Geometry check sheet. Reference: the model listing, model coordinates, mm. A direction names the side the tool comes from. Round coordinates to 2 decimals unless told otherwise and drop trailing zeros. Order: outer loops, then holes, each group sorted by start corner. A loop starts at its lowest first (then second) coordinate and runs counter-clockwise, first axis right, second up. Notation, with made-up numbers: (-5, 29.5) -> (38, 29.5) arc R11 cw to (38, 35.5) -> close; hole circle Ø10 at (-3.5, 23). An arc over 180 degrees is marked (long way). Answer as a JSON object with one key per item and string values. Group by question number.
from build123d import *

# Parameters (mm, degrees)
F0_R     = 10
F1_DEPTH = 7.5
F2_R     = 10
F3_R     = 10
F4_R     = 15
F5_R     = 15


with BuildPart() as f1:
    # F0 (on Front) → F1 (new body, symmetric)
    with BuildSketch(Plane.XZ):
        with BuildLine():
            ThreePointArc((-19.027325, -11.591323), (-14.510885, -6.560614), (-12.878518, 0))
            ThreePointArc((-12.878518, 0), (-14.510885, 6.560614), (-19.027325, 11.591323))
            ThreePointArc((-19.027325, 11.591323), (-40.878518, 0), (-19.027325, -11.591323))
        make_face()
        with Locations((-26.878518, 0)):
            Circle(F0_R, mode=Mode.SUBTRACT)
        with BuildLine():
            Line((54.121482, 0), (-12.878518, 0))
            ThreePointArc((-12.878518, 0), (-14.510885, -6.560614), (-19.027325, -11.591323))
            Line((-19.027325, -11.591323), (63.640685, -21.482518))
            ThreePointArc((63.640685, -21.482518), (56.607871, -11.748551), (54.121482, 0))
        make_face()
        with BuildLine():
            ThreePointArc((-19.027325, 11.591323), (-14.510885, 6.560614), (-12.878518, 0))
            Line((-12.878518, 0), (54.121482, 0))
            ThreePointArc((54.121482, 0), (56.607871, 11.748551), (63.640685, 21.482518))
            Line((63.640685, 21.482518), (-19.027325, 11.591323))
        make_face()
        with BuildLine():
            ThreePointArc((63.640685, 21.482518), (56.607871, 11.748551), (54.121482, 0))
            ThreePointArc((54.121482, 0), (56.607871, -11.748551), (63.640685, -21.482518))
            ThreePointArc((63.640685, -21.482518), (94.870033, -26.513611), (112.121482, 0))
            ThreePointArc((112.121482, 0), (94.870033, 26.513611), (63.640685, 21.482518))
        make_face()
        with BuildLine():
            ThreePointArc((101.121482, 0), (83.121482, -18), (65.121482, 0))
            ThreePointArc((65.121482, 0), (83.121482, 18), (101.121482, 0))
        make_face(mode=Mode.SUBTRACT)
    extrude(amount=F1_DEPTH, both=True)

    # F2
    f2_edges = [f1.edges().sort_by_distance(p)[0] for p in [
        (63.640685, -3.75, 21.482518),
    ]]
    fillet(f2_edges, radius=F2_R)

    # F3
    f3_edges = [f1.edges().sort_by_distance(p)[0] for p in [
        (63.640685, 3.75, -21.482518),
    ]]
    fillet(f3_edges, radius=F3_R)

    # F4
    f4_edges = [f1.edges().sort_by_distance(p)[0] for p in [
        (-19.027325, 0, -11.591323),
    ]]
    fillet(f4_edges, radius=F4_R)

    # F5
    f5_edges = [f1.edges().sort_by_distance(p)[0] for p in [
        (-19.027325, 0, 11.591323),
    ]]
    fillet(f5_edges, radius=F5_R)


solid = f1.part
Item 1: Sectioned sample at B-B, the plane y = -3.75. Enter the section's corners in (x, z).
Item 2: Sectioned sample at D-D, the plane x = 94. Enter the section's corners in (y, z).
Item 3: Sectioned sample at C-C, the plane x = 71. Enter the section's corners in (y, z).
Item 4: Thickness scan on L1, parallel to X at y = 6, z = -3.5; L2, parallel to X at y = -3.25, z = 2.5; L3, parallel to Z at x = -29.5, y = 2.75. Record the ranges inside material, lowest first.
Item 5: Depth check by flat-ended pin: pin 1 Ø6 at (x, y) = (41.5, 0) entering from -Z; pin 2 Ø6 at (x, y) = (94.5, -1.5) entering from +Z; pin 3 Ø12 at (x, z) = (-26.88, 0) entering from +Y; pin 4 Ø6 at (x, y) = (51, 3) entering from -Z. Enter the tip coordinate at first touch or a pass-through.
Item 6: Sectioned sample at A-A, the plane z = 2.5. Enter the section's corners in (x, y), then the cut area to 3 significant figures.
Item 7: Set-up check for faces 4 (the flat face through (22.556, -0.105, -16.567)), 5 (the flat face through (23.61, -0.105, 16.693)), 6 (the cylindrical face through (63.254, -0.105, -21.778)): record each of +Z, -Z, +X, -X, +Y, -Y from which the full face is reachable in a straight line by a thin tool's end or side.
Item 8: Mould release check, pull along X, two halves, no side actions. Record for faces 1 (the cylindrical face through (-18.286, 0.105, 12.145)), 2 (the flat face through (52, -7.5, 0)), 3 (the cylindrical face through (63.254, 0.105, 21.778)): pulls with the +X half, pulls with the -X half, needs draft (parallel to the pull), parting line crosses it, or undercut.
Result:
{
 "1": {"outline": "(-21.79, -13.04) arc R15 cw to (-14.56, -12.13) -> (60.73, -21.13) arc R10 cw to (65.59, -23.1) arc R29 ccw (long way) to (65.59, 23.1) arc R10 cw to (60.73, 21.13) -> (-14.56, 12.13) arc R15 cw to (-21.79, 13.04) arc R14 ccw (long way) to start; hole circle Ø20 at (-26.88, 0); hole circle Ø36 at (83.12, 0)"},
 "2": {"outline": "(-7.5, -26.88) -> (7.5, -26.88) -> (7.5, -14.34) -> (-7.5, -14.34) -> close; (-7.5, 14.34) -> (7.5, 14.34) -> (7.5, 26.88) -> (-7.5, 26.88) -> close"},
 "3": {"outline": "(-7.5, -26.35) -> (7.5, -26.35) -> (7.5, -13.31) -> (-7.5, -13.31) -> close; (-7.5, 13.31) -> (7.5, 13.31) -> (7.5, 26.35) -> (-7.5, 26.35) -> close"},
 "4": {"L1": "x = -40.43 to -36.25, -17.51 to 65.47, 100.78 to 111.91", "L2": "x = -40.65 to -36.56, -17.2 to 65.3, 100.95 to 112.01", "L3": "z = -13.75 to -9.65, 9.65 to 13.75"},
 "5": {"pin 1": "stops at z = -19.19", "pin 2": "stops at z = 27.76", "pin 3": "passes through", "pin 4": "stops at z = -20.33"},
 "6": {"outline": "(-40.65, -7.5) -> (-36.56, -7.5) -> (-36.56, 7.5) -> (-40.65, 7.5) -> close; (-17.2, -7.5) -> (65.3, -7.5) -> (65.3, 7.5) -> (-17.2, 7.5) -> close; (100.95, -7.5) -> (112.01, -7.5) -> (112.01, 7.5) -> (100.95, 7.5) -> close", "area": "1,460 mm2"},
 "7": {"face 4": "-Z, +Y, -Y", "face 5": "+Z, +Y, -Y", "face 6": "-Z, -X, +Y, -Y"},
 "8": {"face 1": "undercut", "face 2": "needs draft", "face 3": "pulls with the -X half"}
}
